Autodesk Inventor part; units mm, degrees
ref_plane "작업 평면1" through (0, 0, 0) normal (0, 0, 1) x (1, 0, 0)
ref_plane "YZ Plane" through (0, 0, 0) normal (1, 0, 0) x (0, 1, 0)
ref_plane "XZ Plane" through (0, 0, 0) normal (0, 1, 0) x (-1, 0, 0)
ref_plane "작업 평면1" through (0, 0, 0) normal (0, 0, 1) x (1, 0, 0)
sketch "스케치1" plane through (0, 0, 0) normal (0, 0, 1) x (1, 0, 0)
  circle A0 centre (-78.0165, 82.8266) radius 1.55
  circle A1 centre (-62.4602, 82.8266) radius 1.55
  circle A2 centre (-62.4602, 98.3829) radius 1.55
  circle A3 centre (-78.0165, 98.3829) radius 1.55
  circle A4 centre (-70.2383, 101.6047) radius 1.55
  circle A5 centre (-59.2383, 90.6047) radius 1.55
  circle A6 centre (-70.2383, 79.6047) radius 1.55
  circle A7 centre (-81.2383, 90.6047) radius 1.55
  arc A8 (-75.2383, 92.033) -> (-65.2383, 92.033) centre (-70.2383, 90.6047) ccw
  arc A9 (-75.2383, 103.5743) -> (-65.2383, 103.5743) centre (-70.2383, 90.6047) ccw
  line L0 (-65.2383, 95.8047) -> (-65.2383, 103.5743)
  line L1 (-75.2383, 95.8047) -> (-75.2383, 103.5743)
  line L2 (-65.2383, 95.8047) -> (-65.2383, 92.033)
  line L3 (-75.2383, 95.8047) -> (-75.2383, 92.033)
  circle A10 centre (-70.2383, 90.6047) radius 1.5
  circle A11 centre (-62.4602, 98.3829) radius 1.65
  circle A12 centre (-59.2383, 90.6047) radius 1.65
  circle A13 centre (-62.4602, 82.8266) radius 1.65
  circle A14 centre (-70.2383, 79.6047) radius 1.65
  circle A15 centre (-78.0165, 82.8266) radius 1.65
  circle A16 centre (-81.2383, 90.6047) radius 1.65
  circle A17 centre (-78.0165, 98.3829) radius 1.65
  line L4 (-56.3383, 90.6047) -> (-56.3383, 58.6047)
  line L5 (-84.1383, 90.6047) -> (-84.1383, 58.6047)
  arc A18 (-75.2383, 103.5743) -> (-84.1383, 90.6047) centre (-70.2383, 90.6047) ccw
  arc A19 (-56.3383, 90.6047) -> (-65.2383, 103.5743) centre (-70.2383, 90.6047) ccw
  line L6 (-84.1383, 58.6047) -> (-56.3383, 58.6047)
  arc A20 (-56.3383, 90.6047) -> (-65.2383, 103.5743) centre (-70.2383, 90.6047) ccw
  arc A21 (-75.2383, 103.5743) -> (-84.1383, 90.6047) centre (-70.2383, 90.6047) ccw
  point P0 (-52.7957, 62.4635)
  point P1 (-70.2383, 90.6047)
  point P2 (-85.25, 10.6344)
  point P3 (-75.25, 10.6344)
  point P4 (-94.15, -2.3352)
  point P5 (-66.35, -2.3352)
  point P6 (-88.3823, -54.5283)
  point P7 (-48.1823, -54.5283)
  point P8 (-88.3823, -54.5283)
  point P9 (-82.9823, -51.5283)
  point P10 (-53.5823, -51.5283)
  point P11 (-48.1823, -54.5283)
  point P12 (-84.1383, 90.6047)
  point P13 (-56.3383, 90.6047)
  dimension "d0" = 0.1
  dimension "d1" = 0.1
  dimension "d2" = 0.1
  dimension "d3" = 0.1
  dimension "d4" = 0.1
  dimension "d5" = 0.1
  dimension "d6" = 0.1
  dimension "d7" = 32
  dimension "d8" = 32
  dimension "d19" = 27.8
extrude "돌출1" add sketch "스케치1" along normal blind 6 contours A8 L2 L0 A9 L1 L3 | A9 L4 L6 L5 | A11 | A12 | A13 | A14 | A15 | A16 | A17
sketch "스케치2" plane through (0, 0, 6) normal (0, 0, 1) x (1, 0, 0)
  line L0 (-65.2383, 103.5743) -> (-65.2383, 92.033)
  arc A0 (-75.2383, 92.033) -> (-65.2383, 92.033) centre (-70.2383, 90.6047) ccw
  line L1 (-75.2383, 92.033) -> (-75.2383, 103.5743)
  arc A1 (-75.2383, 103.5743) -> (-84.1383, 90.6047) centre (-70.2383, 90.6047) ccw
  line L2 (-84.1383, 90.6047) -> (-84.1383, 58.6047)
  line L3 (-84.1383, 58.6047) -> (-56.3383, 58.6047)
  line L4 (-56.3383, 58.6047) -> (-56.3383, 90.6047)
  arc A2 (-56.3383, 90.6047) -> (-65.2383, 103.5743) centre (-70.2383, 90.6047) ccw
  line L5 (-84.1383, 58.6047) -> (-56.3383, 58.6047)
  line L6 (-56.3383, 58.6047) -> (-56.3383, 64.6047)
  line L7 (-56.3383, 64.6047) -> (-84.1383, 64.6047)
  line L8 (-84.1383, 64.6047) -> (-84.1383, 58.6047)
  line L9 (-84.1383, 58.6047) -> (-77.1383, 58.6047)
  line L10 (-77.1383, 58.6047) -> (-63.3383, 58.6047)
  line L11 (-63.3383, 58.6047) -> (-56.3383, 58.6047)
  line L12 (-63.3383, 58.6047) -> (-63.3383, 64.6047)
  line L13 (-77.1383, 58.6047) -> (-77.1383, 64.6047)
  point P0 (0, 0)
  point P1 (-56.3383, 61.6047)
  point P2 (-63.3383, 61.6047)
  dimension "d20" = 6
  dimension "d21" = 7
  dimension "d22" = 13.8
  dimension "d23" = 7
extrude "돌출2" cut sketch "스케치2" against normal blind 10 contours L12 L3 L13 L7
sketch "스케치3" plane through (0, 0, 6) normal (0, 0, 1) x (1, 0, 0)
  line L0 (-63.3383, 64.6047) -> (-63.3383, 58.6047)
  line L1 (-63.3383, 58.6047) -> (-56.3383, 58.6047)
  line L2 (-56.3383, 58.6047) -> (-56.3383, 90.6047)
  arc A0 (-56.3383, 90.6047) -> (-65.2383, 103.5743) centre (-70.2383, 90.6047) ccw
  line L3 (-65.2383, 103.5743) -> (-65.2383, 92.033)
  arc A1 (-75.2383, 92.033) -> (-65.2383, 92.033) centre (-70.2383, 90.6047) ccw
  line L4 (-75.2383, 92.033) -> (-75.2383, 103.5743)
  arc A2 (-75.2383, 103.5743) -> (-84.1383, 90.6047) centre (-70.2383, 90.6047) ccw
  line L5 (-84.1383, 90.6047) -> (-84.1383, 58.6047)
  line L6 (-84.1383, 58.6047) -> (-77.1383, 58.6047)
  line L7 (-77.1383, 58.6047) -> (-77.1383, 64.6047)
  line L8 (-77.1383, 64.6047) -> (-63.3383, 64.6047)
  circle A3 centre (-59.8383, 61.6047) radius 1.35
  circle A4 centre (-80.6383, 61.6047) radius 1.35
  point P0 (0, 0)
  dimension "d26" = 2.7
  dimension "d27" = 2.7
  dimension "d30" = 20.8
extrude "돌출3" cut sketch "스케치3" against normal blind 10 contours A3 | A4
fillet "모깎기1" radius 1 2 edges at (-75.2383, 103.5743, 3) (-65.2383, 103.5743, 3)
sketch "스케치5" plane through (0, 0, 6) normal (0, 0, 1) x (1, 0, 0)
  arc A0 (-63.7732, 102.9097) -> (-65.2383, 102.0245) centre (-64.2383, 102.0245) ccw
  line L0 (-65.2383, 102.0245) -> (-65.2383, 92.033)
  arc A1 (-75.2383, 92.033) -> (-65.2383, 92.033) centre (-70.2383, 90.6047) ccw
  line L1 (-75.2383, 92.033) -> (-75.2383, 102.0245)
  arc A2 (-75.2383, 102.0245) -> (-76.7034, 102.9097) centre (-76.2383, 102.0245) ccw
  arc A3 (-76.7034, 102.9097) -> (-84.1383, 90.6047) centre (-70.2383, 90.6047) ccw
  line L2 (-84.1383, 90.6047) -> (-84.1383, 58.6047)
  line L3 (-84.1383, 58.6047) -> (-77.1383, 58.6047)
  line L4 (-77.1383, 58.6047) -> (-77.1383, 64.6047)
  line L5 (-77.1383, 64.6047) -> (-63.3383, 64.6047)
  line L6 (-63.3383, 64.6047) -> (-63.3383, 58.6047)
  line L7 (-63.3383, 58.6047) -> (-56.3383, 58.6047)
  line L8 (-56.3383, 58.6047) -> (-56.3383, 90.6047)
  arc A4 (-56.3383, 90.6047) -> (-63.7732, 102.9097) centre (-70.2383, 90.6047) ccw
  circle A5 centre (-59.8383, 61.6047) radius 1.35
  circle A6 centre (-80.6383, 61.6047) radius 1.35
  circle A7 centre (-62.4602, 98.3829) radius 1.55
  circle A8 centre (-59.2383, 90.6047) radius 1.55
  circle A9 centre (-62.4602, 82.8266) radius 1.55
  circle A10 centre (-70.2383, 79.6047) radius 1.55
  circle A11 centre (-78.0165, 82.8266) radius 1.55
  circle A12 centre (-81.2383, 90.6047) radius 1.55
  circle A13 centre (-78.0165, 98.3829) radius 1.55
  circle A14 centre (-77.1383, 58.6047) radius 0.75
  line L9 (-77.1383, 58.6047) -> (-77.1383, 64.6047)
  circle A15 centre (-77.1383, 64.6047) radius 0.75
  circle A16 centre (-63.3383, 64.6047) radius 0.75
  circle A17 centre (-63.3383, 58.6047) radius 0.75
  point P0 (0, 0)
  point P1 (-77.1383, 59.3547)
  point P2 (-77.8883, 58.6047)
  dimension "d32" = 1.5
  dimension "d33" = 1.5
  dimension "d34" = 1.5
  dimension "d35" = 1.5
extrude "돌출4" cut sketch "스케치5" against normal blind 10 contours A17 L6 L7 | L7 L6 A17 | A16 L5 L6 | L6 L5 A16 | A15 L4 L5 | L5 L4 A15 | A14 L4 L3 picked at (-77.3024, 59.0737)
properties part number "frame_knee_to_pelvis1" material "PMMA 플라스틱"
The listing builds one solid part. Answer for the finished solid, in the listing's coordinates (mm). A direction names the side the tool comes from. Give positions to 0.01 mm unless a question says otherwise; leave off trailing zeros. Order: outer loops, then holes, each group sorted by start corner. A loop starts at its lowest first (then second) coordinate and runs counter-clockwise, first axis right, second up. Notation, with made-up numbers: (0, 74.5) -> (32, 74.5) arc R15 ccw to (32, 79.5) -> close; hole circle Ø7 at (43.25, 34). An arc over 180 degrees is marked (long way). One line per item, written item: value.
1) Find the intervals of material crossed by line 1 (X direction, y = 83, z = 1.6); line 2 (Y direction, x = -59.5, z = 1.75); line 3 (X direction, y = 97.5, z = 1.15), in increasing order.
Reported:
line 1: x = -84.14 to -79.56, -76.48 to -64, -60.92 to -56.34
line 2: y = 58.6 to 60.3, 62.91 to 89.08, 92.13 to 99.43
line 3: x = -82.31 to -79.29, -76.74 to -75.24, -65.24 to -63.73, -61.19 to -58.17
2) Find section C-C, the plane z = 3.5. Count the separate pieces of the cut face and the enclosed holes in it, plus the area to 3 significant figures.
Reported:
separate pieces: 1
enclosed holes: 9
area: 863 mm^2
3) Find section D-D, the plane x = -74.25. Determine the outline of the cut face in (y, z), plus the area to 3 significant figures.
Reported:
outline: (64.6, 0) -> (87.3, 0) -> (87.3, 6) -> (64.6, 6) -> close
area: 136 mm^2
4) Find section A-A, the plane y = 89.5. Determine the outline of the cut face in (x, z), plus the area to 3 significant figures.
Reported:
outline: (-84.14, 0) -> (-82.33, 0) -> (-82.33, 6) -> (-84.14, 6) -> close; (-80.15, 0) -> (-75.32, 0) -> (-75.32, 6) -> (-80.15, 6) -> close; (-65.16, 0) -> (-60.33, 0) -> (-60.33, 6) -> (-65.16, 6) -> close; (-58.15, 0) -> (-56.34, 0) -> (-56.34, 6) -> (-58.15, 6) -> close
area: 79.7 mm^2
5) Flat-ended cylindrical pins translate along their axes: P1, Ø3, axis at x = -71, z = 4.5, coming from the -Y side; P2, Ø1.8, axis at y = 95.5, z = 2, coming from the +X side. Find the tip coordinate at first contact, or state that the pin passes through.
Reported:
P1: stops at y = 64.6
P2: stops at x = -56.92
6) Find section B-B, the plane x = -70. Determine the outline of the cut face in (y, z).
Reported:
outline: (64.6, 0) -> (78.07, 0) -> (78.07, 6) -> (64.6, 6) -> close; (81.14, 0) -> (85.41, 0) -> (85.41, 6) -> (81.14, 6) -> close
7) Determine the mould class of faces 1 (the cylindrical face through (-77.651, 65.152, 3.042)), 2 (the flat face through (-81, 58.605, 3)), 3 (the flat face through (-84.138, 75, 3)), 4 (the cylindrical face through (-60.98, 97.92, 2.96)) for opening direction Y: pulls with the +Y half, pulls with the -Y half, needs draft (parallel to the pull), parting line crosses it, or undercut.
Reported:
face 1: undercut
face 2: pulls with the -Y half
face 3: needs draft
face 4: undercut
8) A tool of negligible diameter and unlimited length cuts with its end or side. For faces 5 (the flat face through (-63.338, 62, 3)), 6 (the cylindrical face through (-81.44, 89.068, 2.958)), from which of +Z, -Z, +X, -X, +Y, -Y can it reach the whole face along a straight path? Write none if from no direction.
Reported:
face 5: +Z, -Z, -Y
face 6: +Z, -Z
